Here's how the part is built. I have some questions about the finished solid (model axes, mm). A direction names the side the tool comes from. Coordinates: 2 decimals unless noted, no trailing zeros. Write each loop counter-clockwise with the first axis right and the second up, starting at its lowest first coordinate (ties: lowest second). Pieces come first, ordered by that corner, then holes.
(1) For pin 1 Ø5 at (x, z) = (-31.5, 17.5) entering from +Y; pin 2 Ø5 at (x, y) = (-17.06, -17.06) entering from +Z; pin 3 Ø3 at (x, z) = (-17.5, 4) entering from -Y; pin 4 Ø5 at (x, z) = (7.5, 7.5) entering from -Y, each with a flat end and sliding along its axis, tell me the tip position at first contact or that it passes through.
(2) Please list where these lines run through material, in increasing order: probe 1 along Y at (x, z) = (0, 18.75); probe 2 along X at (y, z) = (-0.5, 3.25); probe 3 along X at (y, z) = (19, 6.5).
(3) Imagine slicing it at A-A, the plane y = 0. List the corners of the cut face in (x, z) for me.
(4) Imagine slicing it at C-C, the plane z = 18.75. State how many separate pieces and enclosed holes the cut face has, plus the area to 3 significant figures.
(5) Imagine slicing it at D-D, the plane x = 24.13. List the corners of the cut face in (y, z) for me, plus the area to 3 significant figures.
(6) Which directions (+Z, -Z, +X, -X, +Y, -Y) give clear straight access to the entire face, cutting with the end or side of a thin tool? Please do faces 4 (the cylindrical face through (-0.358, 26.857, 10.302)), 5 (the conical face through (9.4, -12.3, 8.3)).
(7) Thinking about a two-plate mould opening in Y: for faces 1 (the flat face through (-8, -10.1, 16.764)), 2 (the cylindrical face through (-31.83, 29.18, 10.02)), 3 (the flat face through (-1, -19, 0)), which applies, released by +Y, released by -Y, zero draft, split by the parting line, or undercut?
```python
from build123d import *

# Parameters (mm, degrees)
SKETCH1_R                = 43.18
BOSS_EXTRUDE1_DEPTH      = 20.32
M5_CLEARANCE_HOLE1_D     = 5.5
M5_CLEARANCE_HOLE1_DEPTH = 20.32
CIRPATTERN1_COUNT        = 8
SKETCH9_R                = 14.4907
SKETCH9_R_2              = 12.7
BOSS_EXTRUDE2_DEPTH      = 3.556


with BuildPart() as part:
    # Sketch1 → Boss-Extrude1 (new body)
    with BuildSketch(Plane.XY):
        Circle(SKETCH1_R)
    extrude(amount=BOSS_EXTRUDE1_DEPTH)

    # Sketch7 → 1 NPT Tapped Hole2 (revolve, cut)
    with BuildSketch(Plane.YZ):
        Polygon((0, 0), (0, 20.32), (14.4907, 20.32), (14.4907, 16.764), (15.22797859, 16.764), (15.7299152, 0), align=None)
    revolve(axis=Axis((0, 0, -6.35), (0, 0, 1)), mode=Mode.SUBTRACT)

    # M5 Clearance Hole1
    with Locations(Plane(origin=(0, 0, 0), x_dir=(-1, 0, 0), z_dir=(0, 0, -1))):
        with Locations((0, 24.13)):
            m5_clearance_hole1 = Hole(M5_CLEARANCE_HOLE1_D / 2, depth=M5_CLEARANCE_HOLE1_DEPTH)

    # CirPattern1: M5 Clearance Hole1 ×8 about axis
    cirpattern1_axis = Axis((0, 0, 0), (0, 0, 1))
    for i in range(1, CIRPATTERN1_COUNT):
        add(m5_clearance_hole1.rotate(cirpattern1_axis, i * 360 / CIRPATTERN1_COUNT), mode=Mode.SUBTRACT)

    # Sketch9 → Boss-Extrude2 (add)
    with BuildSketch(Plane.XY.offset(20.32)):
        Circle(SKETCH9_R)
        Circle(SKETCH9_R_2, mode=Mode.SUBTRACT)
    extrude(amount=-BOSS_EXTRUDE2_DEPTH)


solid = part.part
```
Recorded:
1. pin 1: stops at y = 31.99
1. pin 2: passes through
1. pin 3: stops at y = -40.11
1. pin 4: stops at y = -42.89
2. probe 1: y = -43.18 to -26.88, -21.38 to -12.7, 12.7 to 21.38, 26.88 to 43.18
2. probe 2: x = -43.18 to -26.83, -21.43 to -15.62, 15.62 to 21.43, 26.83 to 43.18
2. probe 3: x = -38.78 to -19.01, -15.11 to 15.11, 19.01 to 38.78
3. outline: (-43.18, 0) - (-26.88, 0) - (-26.88, 20.32) - (-43.18, 20.32) - close; (-21.38, 0) - (-15.73, 0) - (-15.23, 16.76) - (-12.7, 16.76) - (-12.7, 20.32) - (-21.38, 20.32) - close; (12.7, 16.76) - (15.23, 16.76) - (15.73, 0) - (21.38, 0) - (21.38, 20.32) - (12.7, 20.32) - close; (26.88, 0) - (43.18, 0) - (43.18, 20.32) - (26.88, 20.32) - close
4. separate pieces: 1
4. enclosed holes: 9
4. area: 5,160 mm2
5. outline: (-35.81, 0) - (-2.75, 0) - (-2.75, 20.32) - (-35.81, 20.32) - close; (2.75, 0) - (35.81, 0) - (35.81, 20.32) - (2.75, 20.32) - close
5. area: 1,340 mm2
6. face 4: +Z, -Z
6. face 5: -Z
7. face 1: undercut
7. face 2: split by the parting line
7. face 3: zero draft
